Verification items for the finished model (mm, model axes). A direction names the side the tool comes from. Give positions to 0.01 mm unless a question says otherwise; leave off trailing zeros. Use CSV: the item, a comma, the result in double quotes.
from build123d import *

# Parameters (mm, degrees)
F0_W     = 508
F0_H     = 914.4
F1_DEPTH = 25.4
F2_W     = 52.3558772112
F2_H     = 33.1072211266
F3_DEPTH = 2.54
F4_W     = 48.3446559812
F4_H     = 27.2626578808
F5_DEPTH = 2.54


with BuildPart() as f1:
    # F0 (on Top) → F1 (new body)
    with BuildSketch(Plane.XY):
        with Locations((93.2292269563, 41.5309555829)):
            Rectangle(F0_W, F0_H)
    extrude(amount=F1_DEPTH)

    # F2 (on face) → F3 (cut)
    with BuildSketch(Plane(origin=(0, 0, 0), x_dir=(1, 0, 0), z_dir=(0, 0, -1))):
        with Locations((-134.5928344381, 364.0698194504)):
            Rectangle(F2_W, F2_H)
    extrude(amount=-F3_DEPTH, mode=Mode.SUBTRACT)

    # F4 (on face) → F5 (cut)
    with BuildSketch(Plane(origin=(0, 0, 0), x_dir=(1, 0, 0), z_dir=(0, 0, -1))):
        with Locations((-136.5984450532, -451.6562968493)):
            Rectangle(F4_W, F4_H)
    extrude(amount=-F5_DEPTH, mode=Mode.SUBTRACT)


solid = f1.part
(1) Mould release check, pull along Y, two halves, no side actions. Record for faces 3 (the flat face through (90, 498.731, 13)), 4 (the flat face through (90, 48, 25.4)), 5 (the flat face through (-135, -364, 2.54)): released by +Y, released by -Y, zero draft, split by the parting line, or undercut.
Calculated:
face 3,"released by +Y"
face 4,"zero draft"
face 5,"undercut"
(2) Depth check by flat-ended pin: pin 1 Ø0.8 at (y, z) = (-363.5, 2) entering from -X; pin 2 Ø1.3 at (y, z) = (455, 1) entering from -X. Enter the tip coordinate at first touch or a pass-through.
Calculated:
pin 1,"stops at x = -108.41"
pin 2,"stops at x = -112.43"
(3) Tool access check on faces 1 (the flat face through (347.229, 35, 13)), 2 (the flat face through (-137, 451, 2.54)). Record the directions out of +Z, -Z, +X, -X, +Y, -Y that give a thin tool (end or side, any length) a straight path to the whole face; none if there is none.
Calculated:
face 1,"+Z, -Z, +X, +Y, -Y"
face 2,"-Z, -X"
